Model file for the job. Use its own axes, mm. Coordinates: 2 decimals unless noted, no trailing zeros. Order: outer loops, then holes, each group sorted by start corner. A loop starts at its lowest first (then second) coordinate and runs counter-clockwise, first axis right, second up.
Autodesk Inventor part; units mm, degrees
ref_plane "YZ Plane" through (0, 0, 0) normal (1, 0, 0) x (0, 1, 0)
ref_plane "XZ Plane" through (0, 0, 0) normal (0, 1, 0) x (-1, 0, 0)
ref_plane "XY Plane" through (0, 0, 0) normal (0, 0, 1) x (1, 0, 0)
sketch "Sketch1" plane through (0, 0, 0) normal (0, 0, 1) x (1, 0, 0)
  line L0 (-20, -60) -> (20, -60)
  line L1 (20, -60) -> (20, 60)
  line L2 (20, 60) -> (-20, 60)
  line L3 (-20, 60) -> (-20, -60)
  line L4 (-20, -60) -> (20, 60) construction
  line L5 (20, -60) -> (-20, 60) construction
  circle A0 centre (5, 50) radius 5.5
  circle A1 centre (5, -50) radius 5.5
  line L6 (-20, 0) -> (20, 0) construction
  point P0 (0, 0)
  point P1 (0, 0)
  dimension "d0" = 40
  dimension "d1" = 120
  dimension "d12" = 11
  dimension "d13" = 100
  dimension "d15" = 15
extrude "Plate1" add sketch "Sketch1" along normal blind 2
sketch "Sketch2" plane through (0, 0, 0) normal (0, 0, -1) x (-1, 0, 0)
  line L0 (0, 40) -> (200, 40) construction
  line L1 (200, 40) -> (200, 20) construction
  line L2 (200, 20) -> (0, 20) construction
  line L3 (0, 20) -> (0, 40) construction
  line L4 (-20, 60) -> (20, 60)
  line L5 (-20, -60) -> (-20, 60)
  point P0 (0, 0)
  point P1 (-48, 100)
  point P2 (20, 60)
  point P3 (-50, 98)
  dimension "d6" = 200
  dimension "d9" = 20
  dimension "d10" = 20
  dimension "d11" = 20
mark "Mark1"
fillet "Corner Round1" radius 6 2 edges at (20, -60, 1) (20, 60, 1)
equation "\"d2\" = Thickness"
equation "\"BendReliefWidth\" = Thickness"
equation "\"BendReliefDepth\" = 0.5 * Thickness"
equation "\"CornerReliefSize\" = 4 * Thickness"
equation "\"MinimumRemnant\" = 2 * Thickness"
equation "\"TransitionRadius\" = BendRadius"
equation "\"JacobiRadiusSize\" = BendRadius"
equation "\"GapSize\" = Thickness"
properties part number "TRM 023 face damper" material "AISI 304"
Q1. Cut at A-A, the plane y = -50. List the corners of the cut face in (x, z).
Established:
outline: (-20, 0) - (-0.5, 0) - (-0.5, 2) - (-20, 2) - close; (10.5, 0) - (20, 0) - (20, 2) - (10.5, 2) - close
Q2. Mould opens along Y. For faces 1 (the face through (-3, -60, 1)), 2 (the face through (18.289, 58.196, 1.014)), 3 (the face through (4.284, 44.547, 0.986)), 4 (the face through (-20, 1, 1)) say: pulls with the +Y half, pulls with the -Y half, needs draft (parallel to the pull), parting line crosses it, or undercut.
Established:
face 1: pulls with the -Y half
face 2: pulls with the +Y half
face 3: undercut
face 4: needs draft
Q3. Cut at C-C, the plane x = 9. List the corners of the cut face in (y, z), plus the area to 3 significant figures.
Established:
outline: (-60, 0) - (-53.77, 0) - (-53.77, 2) - (-60, 2) - close; (-46.23, 0) - (46.23, 0) - (46.23, 2) - (-46.23, 2) - close; (53.77, 0) - (60, 0) - (60, 2) - (53.77, 2) - close
area: 210 mm2
Q4. Probe line 1 (Y direction, x = 5, z = 0.5); line 2 (Y direction, x = 7, z = 1.1); line 3 (X direction, y = 47, z = 0.3). List the from-to ranges inside material, lowest first.
Established:
line 1: y = -60 to -55.5, -44.5 to 44.5, 55.5 to 60
line 2: y = -60 to -55.12, -44.88 to 44.88, 55.12 to 60
line 3: x = -20 to 0.39, 9.61 to 20
Q5. Cut at B-B, the plane z = 0.6. List the corners of the cut face in (x, y), plus the area to 3 significant figures.
Established:
outline: (-20, -60) - (14, -60) arc R6 ccw to (20, -54) - (20, 54) arc R6 ccw to (14, 60) - (-20, 60) - close; hole circle Ø11 at (5, -50); hole circle Ø11 at (5, 50)
area: 4,590 mm2
